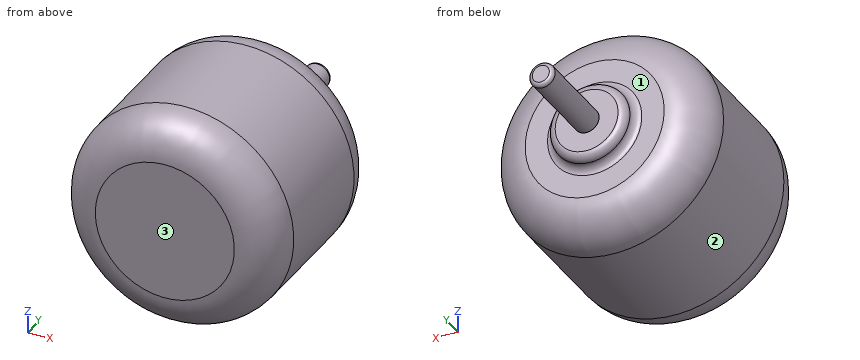
Autodesk Inventor part; units mm, degrees
ref_plane "YZ Plane" through (0, 0, 0) normal (1, 0, 0) x (0, 1, 0)
ref_plane "XZ Plane" through (0, 0, 0) normal (0, 1, 0) x (-1, 0, 0)
ref_plane "XY Plane" through (0, 0, 0) normal (0, 0, 1) x (1, 0, 0)
sketch "Sketch1" plane through (0, 0, 0) normal (0, 1, 0) x (-1, 0, 0)
  point P0 (0, 0)
sketch "Sketch2" plane through (0, 0, 0) normal (0, 1, 0) x (-1, 0, 0)
  circle A0 centre (0, 0) radius 13.85
  dimension "d0" = 27.7
extrude "Extrusion1" add sketch "Sketch2" along normal blind 25
sketch "Sketch3" plane through (0, 25, 0) normal (0, 1, 0) x (1, 0, 0)
  circle A0 centre (0, 0) radius 13.85
  circle A1 centre (0, 0) radius 5
  dimension "d3" = 10
extrude "Extrusion2" add sketch "Sketch3" along normal blind 2 contours A1
sketch "Sketch4" plane through (0, 27, 0) normal (0, 1, 0) x (1, 0, 0)
  circle A0 centre (0, 0) radius 1.585
  dimension "d6" = 3.17
extrude "Extrusion3" add sketch "Sketch4" along normal blind 11.4
fillet "Fillet1" radius 5 2 edges at (13.85, 0, 0) (13.85, 25, 0)
fillet "Fillet2" radius 1 2 edges at (-5, 27, 0) (-5, 25, 0)
fillet "Fillet3" radius 0.5 1 edges at (-1.585, 38.4, 0)
properties part number "Motor"
Geometry: final body of the model. Coordinates: model frame, mm. Face numbers are marked on the shaded views. Round coordinates to 2 decimals unless told otherwise and drop trailing zeros. Order: outer loops, then holes, each group sorted by start corner. A loop starts at its lowest first (then second) coordinate and runs counter-clockwise, first axis right, second up. Notation, with made-up numbers: (14.5, 58) -> (35.5, 58) arc R12 ccw to (35.5, 70) -> close; hole circle Ø3 at (2.5, 54.25). An arc over 180 degrees is marked (long way). Put each result on its own line as item: value. Start each with the question number.
Q1. Section C-C on y = 14. Return the cut outline in (x, z), and give its area (3 significant figures).
Q2. Line query: probe 1 along Y at (x, z) = (6, -1.25); probe 2 along Y at (x, z) = (-1.5, 4); probe 3 along X at (y, z) = (17, 1). Output: solid intervals per line, ascending.
Q3. Pull-direction query (Y, two-part tool) for the marked faces 1, 2 and 3; classes: +Y half, -Y half, draft (parallel to the pull), parting line (faces both ways), or undercut.
Q4. Section D-D on y = 29. Return the cut outline in (x, z) (3 decimals).
Q5. First-contact query: pin 1 (2 mm diameter, centred on x = -8.5, y = 8, fed in from -Z); pin 2 (5 mm diameter, centred on x = 8.5, y = 10.5, fed in from +Z); pin 3 (1.5 mm diameter, centred on x = 2.5, y = 31, fed in from +Z); pin 4 (2 mm diameter, centred on x = -7.5, z = -9.5, fed in from -Y). Flat tips, straight axial feed; report the tip coordinate or a pass-through.
Ans:
1. outline: circle Ø27.7 at (0, 0)
1. area: 603 mm2
2. probe 1: y = 0 to 25
2. probe 2: y = 0 to 26.96
2. probe 3: x = -13.81 to 13.81
3. face 1: +Y half
3. face 2: draft
3. face 3: -Y half
4. outline: circle Ø3.17 at (0, 0)
5. pin 1: stops at z = -11.64
5. pin 2: stops at z = 12.48
5. pin 3: passes through
5. pin 4: stops at y = 0.54
